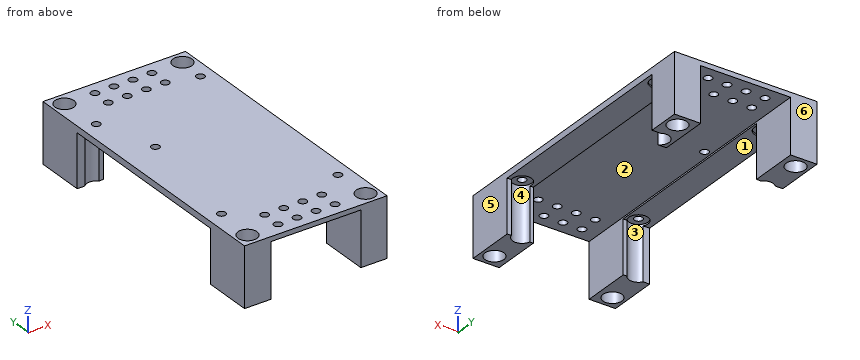
```python
from build123d import *

# Parameters (mm, degrees)
ESQUISSE1_W                  = 60
ESQUISSE1_H                  = 121.051019192
ESQUISSE1_R                  = 4
ESQUISSE1_R_2                = 1.7
BOSS_EXTRU_1_DEPTH           = 25
ESQUISSE2_W                  = 22.3
ESQUISSE2_H                  = 80
ENL_V_MAT_EXTRU_1_DEPTH      = 1
ENL_V_MAT_EXTRU_1_DEPTH_BACK = 61
ESQUISSE3_R                  = 4
ENL_V_MAT_EXTRU_2_DEPTH      = 23
ESQUISSE4_W                  = 37.857644836
ESQUISSE4_H                  = 23
ENL_V_MAT_EXTRU_3_DEPTH      = 142
ESQUISSE5_R                  = 1.7
ENL_V_MAT_EXTRU_4_DEPTH      = 5
ESQUISSE6_W                  = 3.767049496
ESQUISSE6_H                  = 22.3
ENL_V_MAT_EXTRU_5_DEPTH      = 7


with BuildPart() as part:
    # Esquisse1 → Boss.-Extru.1 (new body)
    with BuildSketch(Plane.XY):
        with Locations((-13.883911806, 6.527624962)):
            Rectangle(ESQUISSE1_W, ESQUISSE1_H)
        with Locations((-38.733325391, -48.472375038)):
            Circle(ESQUISSE1_R, mode=Mode.SUBTRACT)
        with Locations((10.965501778, -48.472375038)):
            Circle(ESQUISSE1_R, mode=Mode.SUBTRACT)
        with Locations((10.965501778, 61.527624962)):
            Circle(ESQUISSE1_R, mode=Mode.SUBTRACT)
        with Locations((-38.733325391, 61.527624962)):
            Circle(ESQUISSE1_R, mode=Mode.SUBTRACT)
        with Locations((10.486674609, -32.532375038)):
            Circle(ESQUISSE1_R_2, mode=Mode.SUBTRACT)
        with Locations((10.486674609, 50.067624962)):
            Circle(ESQUISSE1_R_2, mode=Mode.SUBTRACT)
        with Locations((-30.013325391, 19.323966875)):
            Circle(ESQUISSE1_R_2, mode=Mode.SUBTRACT)
        with Locations((-37.713325391, -31.392375038)):
            Circle(ESQUISSE1_R_2, mode=Mode.SUBTRACT)
        with Locations((-37.713325391, 43.847624962)):
            Circle(ESQUISSE1_R_2, mode=Mode.SUBTRACT)
    extrude(amount=BOSS_EXTRU_1_DEPTH)

    # Esquisse2 → Enlèv. mat.-Extru.1 (cut, two sides)
    with BuildSketch(Plane(origin=(16.116088194, 0, 0), x_dir=(0, 0, -1), z_dir=(1, 0, 0))) as enl_v_mat_extru_1_sk:
        with Locations((-11.15, 6.527624962)):
            Rectangle(ESQUISSE2_W, ESQUISSE2_H)
    extrude(amount=ENL_V_MAT_EXTRU_1_DEPTH, mode=Mode.SUBTRACT)
    extrude(enl_v_mat_extru_1_sk.sketch, amount=-ENL_V_MAT_EXTRU_1_DEPTH_BACK, mode=Mode.SUBTRACT)

    # Esquisse3 → Enlèv. mat.-Extru.2 (cut)
    with BuildSketch(Plane(origin=(0, 0, 0), x_dir=(-1, 0, 0), z_dir=(0, 0, -1))):
        with Locations((-10.486674609, -32.532375038)):
            Circle(ESQUISSE3_R)
        with Locations((37.713325391, -31.392375038)):
            Circle(ESQUISSE3_R)
        with Locations((-10.486674609, 50.067624962)):
            Circle(ESQUISSE3_R)
        with Locations((37.713325391, 43.847624962)):
            Circle(ESQUISSE3_R)
    extrude(amount=-ENL_V_MAT_EXTRU_2_DEPTH, mode=Mode.SUBTRACT)

    # Esquisse4 → Enlèv. mat.-Extru.3 (cut)
    with BuildSketch(Plane.XZ.offset(53.997884634)):
        with Locations((-13.831213491, 11.5)):
            Rectangle(ESQUISSE4_W, ESQUISSE4_H)
    extrude(amount=-ENL_V_MAT_EXTRU_3_DEPTH, mode=Mode.SUBTRACT)

    # Esquisse5 → Enlèv. mat.-Extru.4 (cut)
    with BuildSketch(Plane.XY.offset(25)):
        with Locations((-9.883911806, 61.527624962)):
            Circle(ESQUISSE5_R)
        with Locations((-1.883911806, 61.527624962)):
            Circle(ESQUISSE5_R)
        with Locations((-1.883911806, 53.527624962)):
            Circle(ESQUISSE5_R)
        with Locations((-9.883911806, 53.527624962)):
            Circle(ESQUISSE5_R)
        with Locations((-17.883911806, 53.527624962)):
            Circle(ESQUISSE5_R)
        with Locations((-25.883911806, 53.527624962)):
            Circle(ESQUISSE5_R)
        with Locations((-25.883911806, 61.527624962)):
            Circle(ESQUISSE5_R)
        with Locations((-17.883911806, 61.527624962)):
            Circle(ESQUISSE5_R)
        with Locations((-17.883911806, -48.472375038)):
            Circle(ESQUISSE5_R)
        with Locations((-25.883911806, -48.472375038)):
            Circle(ESQUISSE5_R)
        with Locations((-25.883911806, -40.472375038)):
            Circle(ESQUISSE5_R)
        with Locations((-17.883911806, -40.472375038)):
            Circle(ESQUISSE5_R)
        with Locations((-9.883911806, -40.472375038)):
            Circle(ESQUISSE5_R)
        with Locations((-1.883911806, -40.472375038)):
            Circle(ESQUISSE5_R)
        with Locations((-1.883911806, -48.472375038)):
            Circle(ESQUISSE5_R)
        with Locations((-9.883911806, -48.472375038)):
            Circle(ESQUISSE5_R)
    extrude(amount=-ENL_V_MAT_EXTRU_4_DEPTH, mode=Mode.SUBTRACT)

    # Esquisse6 → Enlèv. mat.-Extru.5 (cut)
    with BuildSketch(Plane.XZ.offset(-46.527624962)):
        with Locations((14.232563446, 11.15)):
            Rectangle(ESQUISSE6_W, ESQUISSE6_H)
    extrude(amount=-ENL_V_MAT_EXTRU_5_DEPTH, mode=Mode.SUBTRACT)


solid = part.part
```
Work out the finished part from the listing and answer in its coordinate system (mm). Face numbers are marked on the shaded views. A direction names the side the tool comes from. Give positions to 0.01 mm unless a question says otherwise; leave off trailing zeros. Order: outer loops, then holes, each group sorted by start corner. A loop starts at its lowest first (then second) coordinate and runs counter-clockwise, first axis right, second up.
1. Section B-B, the plane x = -2 is taken. Determine the outline of the cut face in (y, z), and give its area (3 significant figures).
Result sheet:
outline: (-54, 23) - (-50.17, 23) - (-50.17, 25) - (-54, 25) - close; (-46.78, 23) - (-42.17, 23) - (-42.17, 25) - (-46.78, 25) - close; (-38.78, 23) - (51.83, 23) - (51.83, 25) - (-38.78, 25) - close; (55.22, 23) - (59.83, 23) - (59.83, 25) - (55.22, 25) - close; (63.22, 23) - (67.05, 23) - (67.05, 25) - (63.22, 25) - close
area: 215 mm2
2. Section D-D, the plane x = -17.5 is taken. Determine the outline of the cut face in (y, z), and give its area (3 significant figures).
Result sheet:
outline: (-54, 23) - (-50.13, 23) - (-50.13, 25) - (-54, 25) - close; (-46.82, 23) - (-42.13, 23) - (-42.13, 25) - (-46.82, 25) - close; (-38.82, 23) - (51.87, 23) - (51.87, 25) - (-38.82, 25) - close; (55.18, 23) - (59.87, 23) - (59.87, 25) - (55.18, 25) - close; (63.18, 23) - (67.05, 23) - (67.05, 25) - (63.18, 25) - close
area: 216 mm2
3. Straight lines are drawn through the part: L1, parallel to Y at x = -37, z = 22.5; L2, parallel to X at y = -45, z = 6.5; L3, parallel to Y at x = -36.5, z = 8.25. For each, find the intervals that lie inside material, in ascending order.
Result sheet:
L1: y = -54 to -52.08, -44.87 to -35.33, -27.46 to 39.91, 47.78 to 57.92, 65.13 to 67.05
L2: x = -43.88 to -40.72, -36.75 to -32.76, 5.1 to 8.98, 12.95 to 16.12
L3: y = -54 to -51.79, -45.15 to -35.2, 47.66 to 58.21, 64.85 to 67.05
4. The mould has two halves that part along X. Classify the marked faces 4, 5 and 6: released by +X, released by -X, zero draft, split by the parting line, or undercut.
Result sheet:
face 4: undercut
face 5: released by +X
face 6: zero draft
5. Section C-C, the plane y = 24 is taken. Determine the outline of the cut face in (x, z).
Result sheet:
outline: (-43.88, 22.3) - (-32.76, 22.3) - (-32.76, 23) - (5.1, 23) - (5.1, 22.3) - (16.12, 22.3) - (16.12, 25) - (-43.88, 25) - close
6. For the marked faces 1, 2 and 3, determine the directions among +Z, -Z, +X, -X, +Y, -Y from which every point of the face is accessible in a straight line to the end or side of a thin tool.
Result sheet:
face 1: -Z, +X, -X
face 2: -Z, +Y, -Y
face 3: -Z
7. Section A-A, the plane z = 9.25 is taken. Determine the outline of the cut face in (x, y).
Result sheet:
outline: (-43.88, -54) - (-32.76, -54) - (-32.76, -33.47) - (-34.3, -33.47) arc R4 cw to (-41.13, -33.47) - (-43.88, -33.47) - close; (-43.88, 46.53) - (-40.68, 46.53) arc R4 cw to (-34.74, 46.53) - (-32.76, 46.53) - (-32.76, 67.05) - (-43.88, 67.05) - close; (5.1, -54) - (16.12, -54) - (16.12, -33.47) - (14.37, -33.47) arc R4 cw to (6.6, -33.47) - (5.1, -33.47) - close; (5.1, 46.53) - (8.62, 46.53) arc R4 cw (long way) to (12.49, 53.53) - (16.12, 53.53) - (16.12, 67.05) - (5.1, 67.05) - close; hole circle Ø8 at (-38.73, -48.47); hole circle Ø8 at (-38.73, 61.53); hole circle Ø8 at (10.97, -48.47); hole circle Ø8 at (10.97, 61.53)
8. Each of these flat-tipped pins is pushed along its axis until it touches: P1, Ø4.5, axis at x = -9.88, y = 61.53, coming from the -Z side; P2, Ø3, axis at x = -9.88, y = 53.53, coming from the -Z side; P3, Ø1.5, axis at x = 6.5, y = -11.5, coming from the -Z side. Where does it stop, or does it pass through?
Result sheet:
P1: stops at z = 23
P2: passes through
P3: stops at z = 22.3
